```python
from build123d import *

# Parameters (mm, degrees)
F0_W     = 50
F0_H     = 40
F1_DEPTH = 6
F2_W     = 50
F2_H     = 40
F2_W_2   = 46
F2_H_2   = 36
F3_DEPTH = 20
F5_DEPTH = 2


with BuildPart() as f1:
    # F0 (on Top) → F1 (new body)
    with BuildSketch(Plane.XY):
        Rectangle(F0_W, F0_H)
    extrude(amount=F1_DEPTH)

    # F2 (on face) → F3 (join)
    with BuildSketch(Plane.XY.offset(6)):
        Rectangle(F2_W, F2_H)
        Rectangle(F2_W_2, F2_H_2, mode=Mode.SUBTRACT)
    extrude(amount=F3_DEPTH)

    # F4 (on face) → F5 (join)
    with BuildSketch(Plane.XY.offset(6)):
        Polygon((-12, 7), (-12, 12), (-7, 12), (-7, 14), (-14, 14), (-14, 7), align=None)
        Polygon((7, 12), (12, 12), (12, 7), (14, 7), (14, 14), (7, 14), align=None)
        Polygon((14, -7), (12, -7), (12, -12), (7, -12), (7, -14), (14, -14), align=None)
        Polygon((-7, -12), (-12, -12), (-12, -7), (-14, -7), (-14, -14), (-7, -14), align=None)
    extrude(amount=F5_DEPTH)


solid = f1.part
```
The model under review builds one solid part; all positions refer to its coordinate system, in mm. A direction names the side the tool comes from. Give positions to 0.01 mm unless a question says otherwise; leave off trailing zeros. Write each loop counter-clockwise with the first axis right and the second up, starting at its lowest first coordinate (ties: lowest second). Pieces come first, ordered by that corner, then holes.
(1) For P1, Ø5.5, axis at x = 11, y = -12, coming from the +Z side, flat-tipped, find the tip position at first contact; note if it passes through.
(2) Consider section A-A, the plane z = 9. Give the boundary of the cut face in (x, y), and give its area (3 significant figures).
(3) Consider section B-B, the plane y = -15. Give the boundary of the cut face in (x, z).
(4) Consider section D-D, the plane x = -1.5. Give the boundary of the cut face in (y, z), and give its area (3 significant figures).
(5) The part is to be moulded in two halves that separate along Y. For faces 1 (the flat face through (0, 0, 0)), 2 (the flat face through (9, 12, 7)), 3 (the flat face through (0, 20, 13)), say which applies: released by +Y, released by -Y, zero draft, split by the parting line, or undercut.
(6) To check wall thickness, follow L1, parallel to Y at x = -11.5, z = 6.5; L2, parallel to Y at x = 11, z = 13.5; L3, parallel to X at y = 15, z = 12. State the ranges of each line that lie inside material, in increasing order.
(7) Tool access review of faces 4 (the flat face through (-14, -10, 7)), 5 (the flat face through (-25, 0, 13)): name each direction out of +Z, -Z, +X, -X, +Y, -Y from which nothing blocks a thin tool from reaching the whole face with its end or side.
(8) Consider section C-C, the plane x = 10. Give the boundary of the cut face in (y, z).
Returned:
1. P1: stops at z = 8
2. outline: (-25, -20) - (25, -20) - (25, 20) - (-25, 20) - close; hole (-23, -18) - (23, -18) - (23, 18) - (-23, 18) - close
2. area: 344 mm2
3. outline: (-25, 0) - (25, 0) - (25, 26) - (23, 26) - (23, 6) - (-23, 6) - (-23, 26) - (-25, 26) - close
4. outline: (-20, 0) - (20, 0) - (20, 26) - (18, 26) - (18, 6) - (-18, 6) - (-18, 26) - (-20, 26) - close
4. area: 320 mm2
5. face 1: zero draft
5. face 2: undercut
5. face 3: released by +Y
6. L1: y = -20 to -18, -14 to -12, 12 to 14, 18 to 20
6. L2: y = -20 to -18, 18 to 20
6. L3: x = -25 to -23, 23 to 25
7. face 4: +Z
7. face 5: +Z, -Z, -X, +Y, -Y
8. outline: (-20, 0) - (20, 0) - (20, 26) - (18, 26) - (18, 6) - (14, 6) - (14, 8) - (12, 8) - (12, 6) - (-12, 6) - (-12, 8) - (-14, 8) - (-14, 6) - (-18, 6) - (-18, 26) - (-20, 26) - close
